```python
from build123d import *

# Parameters (mm, degrees)
SKETCH_1_R      = 5.05
EXTRUDE_1_DEPTH = 10
FILLET_1_R      = 1


with BuildPart() as part:
    # 草图1 → 凸台-拉伸1 (new body)
    with BuildSketch(Plane.XY):
        with BuildLine():
            Line((39.140934276, -3.548274735), (41.570630213, -3.148020227))
            ThreePointArc((41.570630213, -3.148020227), (44.642381358, -2.351220065), (47.520426727, -1.0142831))
            ThreePointArc((47.520426727, -1.0142831), (47.53125, 0), (47.520426727, 1.0142831))
            ThreePointArc((47.520426727, 1.0142831), (43.486808197, 2.721078851), (39.156174689, 3.375940359))
            ThreePointArc((39.156174689, 3.375940359), (38.965208254, 5.129866986), (38.695718051, 6.873455762))
            ThreePointArc((38.695718051, 6.873455762), (42.709298171, 8.626853835), (46.163723236, 11.319469227))
            ThreePointArc((46.163723236, 11.319469227), (45.911661931, 12.301992738), (45.638691669, 13.27891371))
            ThreePointArc((45.638691669, 13.27891371), (41.300764111, 13.88357451), (36.948202731, 13.395271723))
            ThreePointArc((36.948202731, 13.395271723), (36.309793705, 15.040008999), (35.598212175, 16.654437232))
            ThreePointArc((35.598212175, 16.654437232), (39.021220054, 19.386880688), (41.661038295, 22.881818432))
            ThreePointArc((41.661038295, 22.881818432), (41.163269974, 23.765625), (40.646755194, 24.638608295))
            ThreePointArc((40.646755194, 24.638608295), (36.300141203, 24.09992751), (32.222271816, 22.501737457))
            ThreePointArc((32.222271816, 22.501737457), (31.179926719, 23.925199255), (30.074746968, 25.300446327))
            ThreePointArc((30.074746968, 25.300446327), (32.673910276, 28.825723661), (34.319222442, 32.884809526))
            ThreePointArc((34.319222442, 32.884809526), (33.609669193, 33.609669193), (32.884809526, 34.319222442))
            ThreePointArc((32.884809526, 34.319222442), (28.825723661, 32.673910276), (25.300446327, 30.074746968))
            ThreePointArc((25.300446327, 30.074746968), (23.925199255, 31.179926719), (22.501737457, 32.222271816))
            ThreePointArc((22.501737457, 32.222271816), (24.09992751, 36.300141203), (24.638608295, 40.646755194))
            ThreePointArc((24.638608295, 40.646755194), (23.765625, 41.163269974), (22.881818432, 41.661038295))
            ThreePointArc((22.881818432, 41.661038295), (19.386880688, 39.021220054), (16.654437232, 35.598212175))
            ThreePointArc((16.654437232, 35.598212175), (15.040008999, 36.309793705), (13.395271723, 36.948202731))
            ThreePointArc((13.395271723, 36.948202731), (13.88357451, 41.300764111), (13.27891371, 45.638691669))
            ThreePointArc((13.27891371, 45.638691669), (12.301992738, 45.911661931), (11.319469227, 46.163723236))
            ThreePointArc((11.319469227, 46.163723236), (8.626853835, 42.709298171), (6.873455762, 38.695718051))
            ThreePointArc((6.873455762, 38.695718051), (5.129866986, 38.965208254), (3.375940359, 39.156174689))
            ThreePointArc((3.375940359, 39.156174689), (2.721078851, 43.486808197), (1.0142831, 47.520426727))
            ThreePointArc((1.0142831, 47.520426727), (0, 47.53125), (-1.0142831, 47.520426727))
            ThreePointArc((-1.0142831, 47.520426727), (-2.721078851, 43.486808197), (-3.375940359, 39.156174689))
            ThreePointArc((-3.375940359, 39.156174689), (-5.129866986, 38.965208254), (-6.873455762, 38.695718051))
            ThreePointArc((-6.873455762, 38.695718051), (-8.626853835, 42.709298171), (-11.319469227, 46.163723236))
            ThreePointArc((-11.319469227, 46.163723236), (-12.301992738, 45.911661931), (-13.27891371, 45.638691669))
            ThreePointArc((-13.27891371, 45.638691669), (-13.88357451, 41.300764111), (-13.395271723, 36.948202731))
            ThreePointArc((-13.395271723, 36.948202731), (-15.040008999, 36.309793705), (-16.654437232, 35.598212175))
            ThreePointArc((-16.654437232, 35.598212175), (-19.386880688, 39.021220054), (-22.881818432, 41.661038295))
            ThreePointArc((-22.881818432, 41.661038295), (-23.765625, 41.163269974), (-24.638608295, 40.646755194))
            ThreePointArc((-24.638608295, 40.646755194), (-24.09992751, 36.300141203), (-22.501737457, 32.222271816))
            ThreePointArc((-22.501737457, 32.222271816), (-23.925199255, 31.179926719), (-25.300446327, 30.074746968))
            ThreePointArc((-25.300446327, 30.074746968), (-28.825723661, 32.673910276), (-32.884809526, 34.319222442))
            ThreePointArc((-32.884809526, 34.319222442), (-33.609669193, 33.609669193), (-34.319222442, 32.884809526))
            ThreePointArc((-34.319222442, 32.884809526), (-32.673910276, 28.825723661), (-30.074746968, 25.300446327))
            ThreePointArc((-30.074746968, 25.300446327), (-31.179926719, 23.925199255), (-32.222271816, 22.501737457))
            ThreePointArc((-32.222271816, 22.501737457), (-36.300141203, 24.09992751), (-40.646755194, 24.638608295))
            ThreePointArc((-40.646755194, 24.638608295), (-41.163269974, 23.765625), (-41.661038295, 22.881818432))
            ThreePointArc((-41.661038295, 22.881818432), (-39.021220054, 19.386880688), (-35.598212175, 16.654437232))
            ThreePointArc((-35.598212175, 16.654437232), (-36.309793705, 15.040008999), (-36.948202731, 13.395271723))
            ThreePointArc((-36.948202731, 13.395271723), (-41.300764111, 13.88357451), (-45.638691669, 13.27891371))
            ThreePointArc((-45.638691669, 13.27891371), (-45.679019155, 13.13951809), (-45.718920881, 13))
            Line((-45.718920881, 13), (-100.75, 13))
            ThreePointArc((-100.75, 13), (-113.75, 0), (-100.75, -13))
            Line((-100.75, -13), (-37.089122254, -13))
            ThreePointArc((-37.089122254, -13), (4.835934322, -39.002778475), (39.140934276, -3.548274735))
        make_face()
        with Locations((24.375, 0)):
            Circle(SKETCH_1_R, mode=Mode.SUBTRACT)
        Circle(SKETCH_1_R, mode=Mode.SUBTRACT)
        with Locations((-24.375, 0)):
            Circle(SKETCH_1_R, mode=Mode.SUBTRACT)
        with Locations((-100.75, 0)):
            Circle(SKETCH_1_R, mode=Mode.SUBTRACT)
    extrude(amount=EXTRUDE_1_DEPTH)

    # 圆角1
    fillet_1_edges = [part.edges().sort_by_distance(p)[0] for p in [
        (-73.234460441, 13, 10),
        (-113.75, 0, 10),
        (-68.919561127, -13, 10),
        (-68.919561127, -13, 0),
        (-113.75, 0, 0),
        (-73.234460441, 13, 0),
        (4.835934322, -39.002778475, 10),
        (4.835934322, -39.002778475, 0),
        (-37.089122254, -13, 5),
    ]]
    fillet(fillet_1_edges, radius=FILLET_1_R)


solid = part.part
```
Model file for the job. Use its own axes, mm. A direction names the side the tool comes from. Round coordinates to 2 decimals unless told otherwise and drop trailing zeros. Use CSV: the item, a comma, the result in double quotes. Start each with the question number.
Item 1: Pin check, flat tips, straight feed: P1, Ø13, axis at x = 0, y = 0, coming from the -Z side; P2, Ø4, axis at y = 27, z = 6.5, coming from the -X side; P3, Ø4, axis at x = -65, z = 4.5, coming from the +Y side; P4, Ø6, axis at x = -41, z = 7.5, coming from the -Y side. Stop position of each tip, or through.
Item 2: Two-plate mould, pull along Y, no slides. Class faces 1 (the face through (2.738, 43.428, 4.93)), 2 (the face through (43.546, 2.704, 4.93)), 3 (the face through (-70, -13, 5)): released by +Y, released by -Y, zero draft, split by the parting line, or undercut.
Item 3: Drill centre lines: L1, parallel to Y at x = -100.75, z = 7.5; L2, parallel to Y at x = 0, z = 7; L3, parallel to X at y = -2, z = 1.5. Where is each one in solid material? Low to high. Write a range as [from, to].
Item 4: Band-saw the part on A-A (z = 4.75). State how many separate pieces and enclosed holes the cut face has, and give its area (3 significant figures).
Item 5: Tool access for faces 4 (the face through (41.362, 13.883, 4.93)), 5 (the face through (28.879, 32.704, 4.93)), 6 (the face through (32.644, 28.772, 4.93)), 7 (the face through (-39.064, 19.431, 4.93)): list every direction of +Z, -Z, +X, -X, +Y, -Y with a clear straight run to the whole face (end or side of a thin tool).
Checked values:
1,P1,"stops at z = 0"
1,P2,"stops at x = -32.77"
1,P3,"stops at y = 13"
1,P4,"stops at y = -13"
2,face 1,"released by +Y"
2,face 2,"undercut"
2,face 3,"released by -Y"
3,L1,"y = [-13, -5.05], [5.05, 13]"
3,L2,"y = [-39.3, -5.05], [5.05, 47.53]"
3,L3,"x = [-113.6, -105.39], [-96.11, -29.01], [-19.74, -4.64], [4.64, 19.74], [29.01, 45.54]"
4,separate pieces,"1"
4,enclosed holes,"4"
4,area,"6,890 mm²"
5,face 4,"+Z, -Z"
5,face 5,"+Z, -Z, +Y"
5,face 6,"+Z, -Z, +X"
5,face 7,"+Z, -Z, -X"
